Read the model definition and answer for the solid it produces. Units are mm, in the model's axes. A direction names the side the tool comes from. Coordinates: 2 decimals unless noted, no trailing zeros. Write each loop counter-clockwise with the first axis right and the second up, starting at its lowest first coordinate (ties: lowest second). Pieces come first, ordered by that corner, then holes.
Item 1: A tool of negligible diameter and unlimited length cuts with its end or side. For faces 1 (the face through (0.551, -0.854, -0.502)), 2 (the face through (0, -1, -1)), 3 (the face through (6.32, 1.67, 0.53)), from which of +Z, -Z, +X, -X, +Y, -Y can it reach the whole face along a straight path? Write none if from no direction.
Item 2: Section B-B (z = 2.5) is taken. Give the vertices of the cut face in (x, y), then the cut area to 3 significant figures.
Item 3: Straight lines are drawn through the part: probe 1 along Y at (x, z) = (7.5, 1); probe 2 along Y at (x, z) = (5.5, 0.5); probe 3 along X at (y, z) = (-2, -1.25). For each, find the intervals that lie inside material, in ascending order.
Item 4: Each of these flat-tipped pins is pushed along its axis until it touches: P1, Ø3, axis at x = 8, y = -2, coming from the +Z side; P2, Ø1, axis at x = 2, z = -2, coming from the -Y side; P3, Ø1, axis at y = 2.5, z = -1, coming from the +X side. Where does it stop, or does it pass through?
Item 5: Determine the mould class of faces 4 (the face through (0.55, 0.86, -0.49)), 5 (the face through (1.66, -0.72, -3.25)), 6 (the face through (1.854, -1.4, -1.4)) for opening direction Z: released by +Z, released by -Z, zero draft, split by the parting line, or undercut.
Item 6: Section A-A (x = 7.75) is taken. Give the vertices of the cut face in (y, z).
from build123d import *

# Parameters (mm, degrees)
HEX_2_DEPTH = 1.1176


with BuildPart() as part:
    # BodySke → BaseBody (revolve)
    with BuildSketch(Plane.XY):
        with BuildLine():
            Line((11.3792, 0), (11.3792, 1.28016))
            Line((11.3792, 1.28016), (10.90676, 1.7526))
            Line((10.90676, 1.7526), (1.8542, 1.7526))
            Line((1.8542, 1.7526), (1.8542, 3.3274))
            Line((1.8542, 3.3274), (1.4732, 3.3274))
            ThreePointArc((1.4732, 3.3274), (0.616396771, 2.601989501), (0, 1.6637))
            Line((0, 1.6637), (0, 0))
            Line((0, 0), (11.3792, 0))
        make_face()
    revolve(axis=Axis((0, 0, 0), (1, 0, 0)))

    # Sketch2 → PreBroach (revolve, cut)
    with BuildSketch(Plane.XY):
        Polygon((0, 0.9906), (1.1176, 0.9906), (1.689523177, 0), (0, 0), align=None)
    revolve(axis=Axis((0, 0, 0), (1, 0, 0)), mode=Mode.SUBTRACT)

    # Sketch3 → Hex 2 (cut)
    with BuildSketch(Plane(origin=(0, 0, 0), x_dir=(0, 0, -1), z_dir=(1, 0, 0))):
        Polygon((-0.9906, -0.571923177), (-0.9906, 0.571923177), (0, 1.143846353), (0.9906, 0.571923177), (0.9906, -0.571923177), (0, -1.143846353), align=None)
    extrude(amount=HEX_2_DEPTH, mode=Mode.SUBTRACT)


solid = part.part
Established:
1. face 1: -X
1. face 2: +Z, -Z, -X, +Y, -Y
1. face 3: +X
2. outline: (1.47, -2.2) - (1.85, -2.2) - (1.85, 2.2) - (1.47, 2.2) arc R3.03 ccw to start
2. area: 4.54 mm2
3. probe 1: y = -1.44 to 1.44
3. probe 2: y = -1.68 to 1.68
3. probe 3: x = 0.42 to 1.85
4. P1: stops at z = 1.68
4. P2: stops at y = -2.96
4. P3: stops at x = 1.85
5. face 4: undercut
5. face 5: split by the parting line
5. face 6: zero draft
6. outline: circle Ø3.51 at (0, 0)
